The listing builds one solid part. Answer for the finished solid, in the listing's coordinates (mm). Round coordinates to 2 decimals unless told otherwise and drop trailing zeros. Loops run counter-clockwise (first coordinate to the right, second up) from the corner with the lowest first, then second, coordinate; pieces in that order, holes last. Notation, with made-up numbers: M -23.75,-31.75 L -18.75,-31.75 A25 ccw -18.75,7.25 Z; hole C 48,43 d2. An arc over 180 degrees is marked long. Put each result on its own line as item: value. Start each with the question number.
(1) Section B-B, the plane z = -501 is taken. Determine the outline of the cut face in (x, y).
(2) Flat-ended cylindrical pins translate along their axes: P1, Ø1.9, axis at x = 56.5, y = 2.5, coming from the -Z side; P2, Ø1.9, axis at x = 597, y = 4, coming from the +Z side; P3, Ø3, axis at x = 114, y = 3.5, coming from the -Z side. Find the tip coordinate at first contact, or state that the pin passes through.
(3) Straight lines are drawn through the part: line 1 (Z direction, x = 520, y = 4.5); line 2 (X direction, y = 3.5, z = -521); line 3 (X direction, y = 1.25, z = -490). For each, find the intervals that lie inside material, in ascending order.
(4) Section C-C, the plane x = 125 is taken. Determine the outline of the cut face in (y, z), then the cut area to 3 significant figures.
(5) Section A-A, the plane y = 4.25 is taken. Determine the outline of the cut face in (x, z).
```python
from build123d import *

# Parameters (mm, degrees)
SKETCH1_W           = 609.6
SKETCH1_H           = 609.6
BOSS_EXTRUDE1_DEPTH = 6.35
CUT_EXTRUDE1_DEPTH  = 863.127973389


with BuildPart() as part:
    # Sketch1 → Boss-Extrude1 (new body)
    with BuildSketch(Plane(origin=(0, 0, 0), x_dir=(1, 0, 0), z_dir=(0, 1, 0))):
        with Locations((304.8, 304.8)):
            Rectangle(SKETCH1_W, SKETCH1_H)
    extrude(amount=BOSS_EXTRUDE1_DEPTH)

    # Sketch2 → Cut-Extrude1 (cut, through all)
    with BuildSketch(Plane(origin=(0, 6.35, 0), x_dir=(1, 0, 0), z_dir=(0, 1, 0))):
        Polygon((609.6, 0), (476.25, 0), (476.25, 25.4), (508, 25.4), (508, 101.6), (584.2, 101.6), (584.2, 133.35), (609.6, 133.35), align=None)
        Polygon((0, 133.35), (0, 0), (133.35, 0), (133.35, 25.4), (101.6, 25.4), (101.6, 101.6), (25.4, 101.6), (25.4, 133.35), align=None)
        Polygon((0, 609.6), (133.35, 609.6), (133.35, 584.2), (101.6, 584.2), (101.6, 508), (25.4, 508), (25.4, 476.25), (0, 476.25), align=None)
        Polygon((609.6, 476.25), (609.6, 609.6), (476.25, 609.6), (476.25, 584.2), (508, 584.2), (508, 508), (584.2, 508), (584.2, 476.25), align=None)
    extrude(amount=-CUT_EXTRUDE1_DEPTH, mode=Mode.SUBTRACT)


solid = part.part
```
Recorded:
1. outline: M 25.4,0 L 584.2,0 L 584.2,6.35 L 25.4,6.35 Z
2. P1: stops at z = -508
2. P2: stops at z = -133.35
2. P3: stops at z = -584.2
3. line 1: z = -508 to -101.6
3. line 2: x = 101.6 to 508
3. line 3: x = 25.4 to 584.2
4. outline: M 0,-584.2 L 6.35,-584.2 L 6.35,-25.4 L 0,-25.4 Z
4. area: 3,550 mm²
5. outline: M 0,-476.25 L 25.4,-476.25 L 25.4,-508 L 101.6,-508 L 101.6,-584.2 L 133.35,-584.2 L 133.35,-609.6 L 476.25,-609.6 L 476.25,-584.2 L 508,-584.2 L 508,-508 L 584.2,-508 L 584.2,-476.25 L 609.6,-476.25 L 609.6,-133.35 L 584.2,-133.35 L 584.2,-101.6 L 508,-101.6 L 508,-25.4 L 476.25,-25.4 L 476.25,0 L 133.35,0 L 133.35,-25.4 L 101.6,-25.4 L 101.6,-101.6 L 25.4,-101.6 L 25.4,-133.35 L 0,-133.35 Z
